For this review, take the finished solid that the model builds, in its own axes (mm). Give positions to 0.01 mm unless a question says otherwise; leave off trailing zeros. Write each loop counter-clockwise with the first axis right and the second up, starting at its lowest first coordinate (ties: lowest second). Pieces come first, ordered by that corner, then holes. Notation, with made-up numbers: M -11.5,49 L 24.5,49 A7 ccw 24.5,56 Z; hole C 54.5,68.5 d8. An arc over 180 degrees is marked long. Write item = value, one per line.
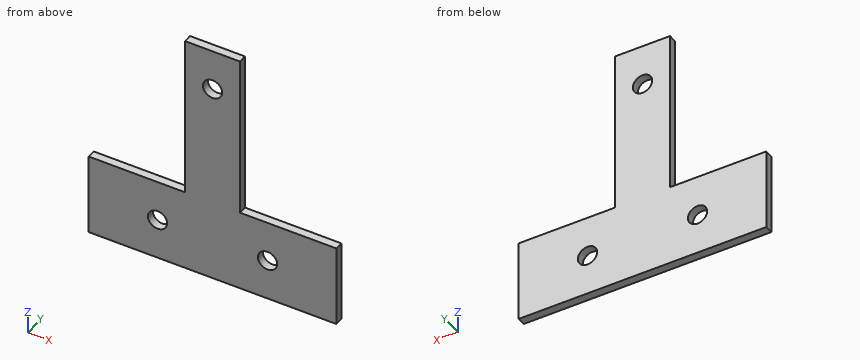
Autodesk Inventor part; units mm, degrees
ref_plane "YZ Plane" through (0, 0, 0) normal (1, 0, 0) x (0, 1, 0)
ref_plane "XZ Plane" through (0, 0, 0) normal (0, 1, 0) x (-1, 0, 0)
ref_plane "XY Plane" through (0, 0, 0) normal (0, 0, 1) x (1, 0, 0)
sketch "Sketch1" plane through (0, 0, 0) normal (0, 1, 0) x (-1, 0, 0)
  line L0 (-10, 0) -> (-10, 60)
  line L1 (-10, 60) -> (10, 60)
  line L2 (10, 60) -> (10, 0)
  line L3 (10, 0) -> (45, 0)
  line L4 (45, 0) -> (45, -30)
  line L5 (45, -30) -> (-45, -30)
  line L6 (-45, -30) -> (-45, 0)
  line L7 (-45, 0) -> (-10, 0)
  point P0 (0, 0)
  point P1 (0, 60)
  dimension "d0" = 20
  dimension "d1" = 30
  dimension "d2" = 60
  dimension "d3" = 90
extrude "Plate1" add sketch "Sketch1" along normal mid plane 3
sketch "Sketch2" plane through (0, 1.5, 0) normal (0, 1, 0) x (1, 0, 0)
  line L0 (10, -60) -> (-10, -60)
  line L1 (45, 30) -> (45, 0)
  line L2 (-45, 0) -> (-45, 30)
  point P0 (0, 0)
  point P1 (0, -45)
  point P2 (20, 15)
  point P3 (-20, 15)
  point P4 (-45, 15)
  dimension "d5" = 15
  dimension "d6" = 25
  dimension "d7" = 25
hole "Hole1" at (0, 1.5, 45) at (20, 1.5, -15) at (-20, 1.5, -15) direction (0, -1, 0) diameter 7 depth 3
equation "\"d13\" = Thickness"
equation "\"d4\" = Thickness"
equation "\"BendRadius\" = Thickness"
equation "\"BendReliefWidth\" = Thickness"
equation "\"BendReliefDepth\" = 0.5 * Thickness"
equation "\"CornerReliefSize\" = 4 * Thickness"
equation "\"MinimumRemnant\" = 2 * Thickness"
equation "\"TransitionRadius\" = BendRadius"
equation "\"JacobiRadiusSize\" = BendRadius"
equation "\"GapSize\" = Thickness"
properties part number "HCMUTE-CDT23-OP_TAMLOT" material "Stainless Steel"
1. We need section A-A, the plane x = 0. Write out the cut boundary in (y, z).
Responses:
outline = M -1.5,-30 L 1.5,-30 L 1.5,41.5 L -1.5,41.5 Z; M -1.5,48.5 L 1.5,48.5 L 1.5,60 L -1.5,60 Z
2. We need section B-B, the plane z = -15. Write out the cut boundary in (x, y).
Responses:
outline = M -45,-1.5 L -23.5,-1.5 L -23.5,1.5 L -45,1.5 Z; M -16.5,-1.5 L 16.5,-1.5 L 16.5,1.5 L -16.5,1.5 Z; M 23.5,-1.5 L 45,-1.5 L 45,1.5 L 23.5,1.5 Z
3. For line 1 along X through (y, z) = (-0.05, -15); line 2 along X through (y, z) = (-0.55, -12); line 3 along Z through (x, y) = (-20, 0.8), list the stretches that pass through material, from the lowest coordinate up. Write a range as from..to.
Responses:
line_1 = -45..-23.5, -16.5..16.5, 23.5..45
line_2 = -45..-21.8, -18.2..18.2, 21.8..45
line_3 = -30..-18.5, -11.5..0
4. We need section C-C, the plane z = 45. Write out the cut boundary in (x, y), then the cut area to 3 significant figures.
Responses:
outline = M -10,-1.5 L -3.5,-1.5 L -3.5,1.5 L -10,1.5 Z; M 3.5,-1.5 L 10,-1.5 L 10,1.5 L 3.5,1.5 Z
area = 39.0 mm2
5. We need section D-D, the plane y = -0.9. Write out the cut boundary in (x, z).
Responses:
outline = M -45,-30 L 45,-30 L 45,0 L 10,0 L 10,60 L -10,60 L -10,0 L -45,0 Z; hole C -20,-15 d7; hole C 0,45 d7; hole C 20,-15 d7
6. Insertion check: P1, Ø0.9, axis at x = 30, y = -0.5, coming from the +Z side; P2, Ø0.9, axis at y = 0, z = 17.5, coming from the -X side. Each pin has a flat end and moves straight along its axis. Give the tip position at first contact, or say it passes through.
Responses:
P1 = 0
P2 = -10
